Autodesk Inventor part; units mm, degrees
ref_plane "YZ Plane" through (0, 0, 0) normal (1, 0, 0) x (0, 1, 0)
ref_plane "XZ Plane" through (0, 0, 0) normal (0, 1, 0) x (-1, 0, 0)
ref_plane "XY Plane" through (0, 0, 0) normal (0, 0, 1) x (1, 0, 0)
sketch "Sketch1" plane through (0, 0, 0) normal (0, 1, 0) x (-1, 0, 0)
  line L0 (-660.4, 0) -> (-660.4, 25.4)
  line L1 (-113.1604, 25.4) -> (-351.652, -111.264)
  line L2 (-351.652, -111.264) -> (-415.4102, 0)
  line L3 (-444.6849, 0) -> (-660.4, 0)
  line L4 (-660.4, 0) -> (-660.4, 25.4)
  line L5 (-660.4, 25.4) -> (-429.9653, 25.4)
  line L6 (-429.9653, 25.4) -> (-415.4102, 0)
  line L7 (-113.1604, 25.4) -> (-100.5318, 3.3619)
  line L8 (-100.5318, 3.3619) -> (-361.0615, -145.9308)
  line L9 (-361.0615, -145.9308) -> (-444.6849, 0)
  line L10 (-660.4, 0) -> (-660.4, 25.4)
  line L11 (-113.1604, 25.4) -> (-351.652, -111.264)
  line L12 (-351.652, -111.264) -> (-415.4102, 0)
  line L13 (-444.6849, 0) -> (-660.4, 0)
  line L14 (-660.4, 0) -> (-660.4, 25.4)
  line L15 (-660.4, 25.4) -> (-429.9653, 25.4)
  line L16 (-429.9653, 25.4) -> (-415.4102, 0)
  line L17 (-113.1604, 25.4) -> (-100.5318, 3.3619)
  line L18 (-100.5318, 3.3619) -> (-361.0615, -145.9308)
  line L19 (-361.0615, -145.9308) -> (-444.6849, 0)
  point P0 (0, 0)
  point P1 (-113.1604, 0)
  point P2 (-113.1604, 0)
  dimension "d0" = 25.4
  dimension "d1" = 25.4
  dimension "d2" = 25.4
  dimension "d3" = 25.4
  dimension "d4" = 25.4
  dimension "d5" = 25.4
extrude "Extrusion1" add sketch "Sketch1" along normal blind 25.4
sketch "Sketch2" plane through (0, 25.4, 0) normal (0, 1, 0) x (1, 0, 0)
  line L0 (660.4, -25.4) -> (660.4, 0)
  line L1 (429.9653, -25.4) -> (660.4, -25.4)
  line L2 (660.4, -12.7) -> (647.7, -12.7)
  circle A0 centre (647.7, -12.7) radius 3.3782
  point P0 (0, 0)
  dimension "d8" = 12.7
  dimension "d9" = 6.7564
extrude "Extrusion2" cut sketch "Sketch2" against normal blind 25.4
sketch "Sketch3" plane through (113.1604, 0, 25.4) normal (-0.8676421, 0, 0.4971894) x (0.4971894, 0, 0.8676421)
  line L0 (-25.4, 0) -> (0, 0)
  line L1 (0, 0) -> (0, 25.4)
  line L2 (-25.4, 25.4) -> (0, 25.4)
  line L3 (-25.4, 0) -> (-25.4, 25.4)
  point P0 (-78.3002, 0)
extrude "Extrusion3" add sketch "Sketch3" along normal blind 63.5
properties part number "bar 3"
Can you work these out from the model? Positions are in its coordinate system, mm. A direction names the side the tool comes from. Coordinates: 2 decimals unless noted, no trailing zeros. Loops run counter-clockwise (first coordinate to the right, second up) from the corner with the lowest first, then second, coordinate; pieces in that order, holes last. Notation, with made-up numbers: (-25.5, 79.5) - (32.5, 79.5) arc R29 cw to (32.5, 99.5) - close; hole circle Ø11 at (-30, 58.5). An arc over 180 degrees is marked (long way). Answer as CSV lines item,"result". Start each with the question number.
1) Suppose I cut it at C-C (x = 496.5). Please give me the cut outline in (y, z), plus the area to 3 significant figures.
2) Suppose I cut it at A-A (y = 10). Please give me the cut outline in (x, z), plus the area to 3 significant figures.
3) Which directions (+Z, -Z, +X, -X, +Y, -Y) give clear straight access to the entire face, cutting with the end or side of a thin tool? Please do faces 1 (the flat face through (51.662, 12.878, 45.798)), 2 (the flat face through (551, 13, 0)), 3 (the flat face through (547, 13, 25.4)).
4) Suppose I cut it at D-D (z = -128.5). Please give me the cut outline in (x, y), plus the area to 3 significant figures.
5) I need wall thicknesses on line 1 (X direction, y = 19.5, z = 12.7); line 2 (Z direction, x = 647.7, y = 14.25); line 3 (Z direction, x = 514.5, y = 24). Which ranges of each line are inside material? Lowest first, please. Write a range as from..to.
6) For pin 1 (6 mm diameter, centred on x = 538, y = 8.5, fed in from -Z); pin 2 (6 mm diameter, centred on x = 595, y = 11, fed in from +Z); pin 3 (6 mm diameter, centred on y = 20.5, z = -97.5, fed in from +X), each with a flat end and sliding along its axis, tell me the tip position at first contact or that it passes through.
7) Suppose I cut it at B-B (z = -42.5). Please give me the cut outline in (x, y).
Check result:
1,outline,"(0, 0) - (25.4, 0) - (25.4, 25.4) - (0, 25.4) - close"
1,area,"645 mm²"
2,outline,"(45.44, 34.93) - (361.06, -145.93) - (444.68, 0) - (660.4, 0) - (660.4, 25.4) - (429.97, 25.4) - (351.65, -111.26) - (113.16, 25.4) - (58.07, 56.97) - close; hole circle Ø6.76 at (647.7, 12.7)"
2,area,"18,700 mm²"
3,face 1,"+Z, -X, +Y, -Y"
3,face 2,"-Z, +X, +Y, -Y"
3,face 3,"+Z, +X, +Y, -Y"
4,outline,"(330.64, 0) - (371.05, 0) - (371.05, 25.4) - (330.64, 25.4) - close"
4,area,"1,030 mm²"
5,line 1,"x = 84.24..135.32, 422.69..644.32, 651.08..660.4"
5,line 2,"z = 0..9.32, 16.08..25.4"
5,line 3,"z = 0..25.4"
6,pin 1,"stops at z = 0"
6,pin 2,"stops at z = 25.4"
6,pin 3,"stops at x = 390.53"
7,outline,"(180.57, 0) - (231.65, 0) - (231.65, 25.4) - (180.57, 25.4) - close; (391.06, 0) - (420.33, 0) - (420.33, 25.4) - (391.06, 25.4) - close"
